from build123d import *

# Parameters (mm, degrees)
BOSS_EXTRUDE1_DEPTH = 14
BOSS_EXTRUDE2_DEPTH = 5


with BuildPart() as part:
    # Sketch1 → Boss-Extrude1 (new body)
    with BuildSketch(Plane.XY):
        Polygon((1.75, 2), (1.75, 7), (-1.75, 7), (-1.75, 2), (-5.25, 2), (-5.25, -2), (5.25, -2), (5.25, 2), align=None)
    extrude(amount=BOSS_EXTRUDE1_DEPTH)

    # Sketch2 → Boss-Extrude2 (add)
    with BuildSketch(Plane.XY.offset(14)):
        with BuildLine():
            Line((-1.75, -2), (-0.75, -2))
            ThreePointArc((-0.75, -2), (0, -2.75), (0.75, -2))
            Line((0.75, -2), (1.75, -2))
            ThreePointArc((1.75, -2), (0, -3.75), (-1.75, -2))
        make_face()
    extrude(amount=-BOSS_EXTRUDE2_DEPTH)


solid = part.part
For this review, take the finished solid that the model builds, in its own axes (mm). A direction names the side the tool comes from. Give positions to 0.01 mm unless a question says otherwise; leave off trailing zeros. Loops run counter-clockwise (first coordinate to the right, second up) from the corner with the lowest first, then second, coordinate; pieces in that order, holes last.
Item 1: Take a section at D-D, the plane y = 4. State the section outline as (x, z) points.
Item 2: For line 1 along Y through (x, z) = (-0.25, 7.25); line 2 along X through (y, z) = (3.75, 10.75); line 3 along Y through (x, z) = (0, 12), list the stretches that pass through material, from the lowest coordinate up.
Item 3: Draft analysis for pull direction X (two halves, no side actions). For faces 5 (the flat face through (-5.25, 0, 7)), 6 (the cylindrical face through (-0.02, -2.75, 11.54)), 7 (the flat face through (0, 2, 0)), 8 (the flat face through (1.75, 4, 7)), state which applies: +X half, -X half, draft (parallel to the pull), parting line (faces both ways), or undercut.
Item 4: Take a section at C-C, the plane z = 5.25. State the section outline as (x, y) points.
Item 5: Take a section at B-B, the plane z = 9.5. State the section outline as (x, y) points, and give its area (3 significant figures).
Item 6: Take a section at A-A, the plane x = 0. State the section outline as (y, z) points, and give its area (3 significant figures).
Item 7: Insertion check: pin 1 (4 mm diameter, centred on y = 5.5, z = 7, fed in from +X); pin 2 (1 mm diameter, centred on x = 4, z = 7, fed in from +Y). Each pin has a flat end and moves straight along its axis. Give the tip position at first contact, or say it passes through.
Item 8: Tool access review of faces 1 (the flat face through (4, 2, 7)), 2 (the flat face through (5.25, 0, 7)), 3 (the flat face through (-1.75, 5, 7)), 4 (the flat face through (0, -3, 9)): name each direction out of +Z, -Z, +X, -X, +Y, -Y from which nothing blocks a thin tool from reaching the whole face with its end or side.
Calculated:
1. outline: (-1.75, 0) - (1.75, 0) - (1.75, 14) - (-1.75, 14) - close
2. line 1: y = -2 to 7
2. line 2: x = -1.75 to 1.75
2. line 3: y = -3.75 to -2.75, -2 to 7
3. face 5: -X half
3. face 6: undercut
3. face 7: draft
3. face 8: +X half
4. outline: (-5.25, -2) - (5.25, -2) - (5.25, 2) - (1.75, 2) - (1.75, 7) - (-1.75, 7) - (-1.75, 2) - (-5.25, 2) - close
5. outline: (-5.25, -2) - (-1.75, -2) arc R1.75 ccw to (1.75, -2) - (5.25, -2) - (5.25, 2) - (1.75, 2) - (1.75, 7) - (-1.75, 7) - (-1.75, 2) - (-5.25, 2) - close; hole (-0.75, -2) arc R0.75 ccw to (0.75, -2) - close
5. area: 63.4 mm2
6. outline: (-3.75, 9) - (-2.75, 9) - (-2.75, 14) - (-3.75, 14) - close; (-2, 0) - (7, 0) - (7, 14) - (-2, 14) - close
6. area: 131 mm2
7. pin 1: stops at x = 1.75
7. pin 2: stops at y = 2
8. face 1: +Z, -Z, +X, +Y
8. face 2: +Z, -Z, +X, +Y, -Y
8. face 3: +Z, -Z, -X, +Y
8. face 4: -Z, +X, -X, -Y
